Geometry check sheet. Reference: the model listing, model coordinates, mm. A direction names the side the tool comes from. Round coordinates to 2 decimals unless told otherwise and drop trailing zeros. Order: outer loops, then holes, each group sorted by start corner. A loop starts at its lowest first (then second) coordinate and runs counter-clockwise, first axis right, second up.
(1) Cross-section at A-A on z = 1.5. Enter the section's corners in (x, y), and give its area (3 significant figures).
(2) Cross-section at D-D on x = 0. Enter the section's corners in (y, z), and give its area (3 significant figures).
(3) Cross-section at C-C on z = -18.5. Enter the section's corners in (x, y), and give its area (3 significant figures).
(4) Gauge pin test, flat ends, axial feed: P1, Ø5, axis at x = 1, z = -5.5, coming from the -Y side; P2, Ø1.1, axis at x = -0.5, z = -30.5, coming from the -Y side; P3, Ø6.5, axis at x = 2, y = 3, coming from the -Z side; P4, Ø1, axis at x = 9.5, y = 4, coming from the +Z side. Record the tip position at first contact, or that the pin passes through.
(5) Thickness scan on L1, parallel to Y at x = 9.5, z = 1.5; L2, parallel to Z at x = -2.25, y = -10.5; L3, parallel to X at y = 0, z = 2. Record the ranges inside material, lowest first.
(6) Draft check along Y on faces 4 (the face through (0, -11.1, 2)), 5 (the face through (0, -7, 5)), 6 (the face through (-0.2, -11.6, -29.5)). Enter one of: pulls with the +Y half, pulls with the -Y half, needs draft (parallel to the pull), parting line crosses it, or undercut.
(7) Set-up check for faces 1 (the face through (-0.2, -11.1, -29.5)), 2 (the face through (-11.2, -1, 2)), 3 (the face through (-0.2, -12.1, -30.5)): record each of +Z, -Z, +X, -X, +Y, -Y from which the full face is reachable in a straight line by a thin tool's end or side.
(8) Cross-section at B-B on y = -1.5. Enter the section's corners in (x, z), and give its area (3 significant figures).
from build123d import *

# Parameters (mm, degrees)
F0_W       = 26.4
F0_H       = 16
F0_W_2     = 22.4
F0_H_2     = 12
F1_DEPTH   = 5
F3_DEPTH   = 32
F4_W       = 26.4
F4_H       = 2
F5_DEPTH   = 5.1
F6_W       = 26.4
F6_H       = 2
F7_DEPTH   = 2
F8_W       = 26.4
F8_H       = 2
F9_DEPTH   = 1
F11_DEPTH  = 26.401
F13_DEPTH  = 2
F14_DEPTH  = 26.4
F14_FACE_W = 22.4
F14_FACE_H = 6
F15_DEPTH  = 31.001
F16_DEPTH  = 25


with BuildPart() as f1:
    # F0 (on Top) → F1 (new body)
    with BuildSketch(Plane.XY):
        Rectangle(F0_W, F0_H)
        Rectangle(F0_W_2, F0_H_2, mode=Mode.SUBTRACT)
    extrude(amount=F1_DEPTH)

    # F2 (on face) → F3 (join)
    with BuildSketch(Plane(origin=(0, 0, 0), x_dir=(1, 0, 0), z_dir=(0, 0, -1))):
        Polygon((13.2, 8), (-13.2, 8), (-13.2, 6), (-11.2, 6), (11.2, 6), (13.2, 6), align=None)
    extrude(amount=F3_DEPTH)

    # F4 (on face) → F5 (join)
    with BuildSketch(Plane.XZ.offset(8)):
        with Locations((0, 4)):
            Rectangle(F4_W, F4_H)
        with Locations((0, -31)):
            Rectangle(F4_W, F4_H)
    extrude(amount=F5_DEPTH)

    # F6 (on face) → F7 (join)
    with BuildSketch(Plane(origin=(0, 0, 3), x_dir=(1, 0, 0), z_dir=(0, 0, -1))):
        with Locations((0, 12.1)):
            Rectangle(F6_W, F6_H)
    extrude(amount=F7_DEPTH)

    # F8 (on face) → F9 (join)
    with BuildSketch(Plane.XY.offset(-30)):
        with Locations((0, -12.1)):
            Rectangle(F8_W, F8_H)
    extrude(amount=F9_DEPTH)

    # F10 (on face) → F11 (cut, through all)
    with BuildSketch(Plane(origin=(-13.2, 0, 0), x_dir=(0, -1, 0), z_dir=(-1, 0, 0))):
        Polygon((11.1, -29), (12.1, -30), (12.1, -31), (6, -31), (6, -32), (13.1, -32), (13.1, -29), align=None)
    extrude(amount=-F11_DEPTH, mode=Mode.SUBTRACT)

    # F12 (on face) → F13 (join, through all)
    with BuildSketch(Plane(origin=(-13.2, 0, 0), x_dir=(0, -1, 0), z_dir=(-1, 0, 0))):
        Polygon((0, 0), (6, 0), (6, -7), (6, -31), (12.1, -31), (12.1, -30), (11.1, -29), (11.1, -30), (8, -30), (8, 3), (11.1, 3), (11.1, 1), (13.1, 1), (13.1, 5), (-8, 5), (-8, 0), align=None)
    extrude(amount=-F13_DEPTH)

    # F12 (on face) → F14 (join, through all)
    with BuildSketch(Plane(origin=(-13.2, 0, 0), x_dir=(0, -1, 0), z_dir=(-1, 0, 0))):
        Polygon((6, -7), (6, 0), (0, 0), align=None)
    extrude(amount=-F14_DEPTH)

    # F14_face (on face) → F15 (cut, through all)
    with BuildSketch(Plane(origin=(0, -3, 0), x_dir=(1, 0, 0), z_dir=(0, 0, 1))):
        Rectangle(F14_FACE_W, F14_FACE_H)
    extrude(amount=-F15_DEPTH, mode=Mode.SUBTRACT)

    # F4 (on face) → F16 (cut)
    with BuildSketch(Plane.XZ.offset(8)):
        with BuildLine():
            ThreePointArc((-10.2, -25.023081), (-9.448807, -27.008746), (-7.571423, -28))
            Line((-7.571423, -28), (7.2, -28))
            ThreePointArc((7.2, -28), (9.32132, -27.12132), (10.2, -25))
            Line((10.2, -25), (10.2, -17.8))
            ThreePointArc((10.2, -17.8), (0, -7.6), (-10.2, -17.8))
            Line((-10.2, -17.8), (-10.2, -25.023081))
        make_face()
    extrude(amount=-F16_DEPTH, mode=Mode.SUBTRACT)


solid = f1.part
Found:
1. outline: (-13.2, -13.1) - (13.2, -13.1) - (13.2, -11.1) - (-13.2, -11.1) - close; (-13.2, -8) - (13.2, -8) - (13.2, 8) - (-13.2, 8) - close; hole (-11.2, -6) - (11.2, -6) - (11.2, 6) - (-11.2, 6) - close
1. area: 206 mm2
2. outline: (-13.1, 1) - (-11.1, 1) - (-11.1, 3) - (-8, 3) - (-8, -7.6) - (-6, -7.6) - (-6, 5) - (-13.1, 5) - close; (-12.1, -31) - (-6, -31) - (-6, -28) - (-8, -28) - (-8, -30) - (-11.1, -30) - (-11.1, -29) - (-12.1, -30) - close; (6, 0) - (8, 0) - (8, 5) - (6, 5) - close
2. area: 60.0 mm2
3. outline: (-13.2, -8) - (-10.2, -8) - (-10.2, -6) - (-13.2, -6) - close; (10.2, -8) - (13.2, -8) - (13.2, -6) - (10.2, -6) - close
3. area: 12.0 mm2
4. P1: stops at y = -8
4. P2: stops at y = -12.1
4. P3: stops at z = 0
4. P4: passes through
5. L1: y = -13.1 to -11.1, -8 to -6, 6 to 8
5. L2: z = -31 to -30, 3 to 5
5. L3: x = -13.2 to -11.2, 11.2 to 13.2
6. face 4: undercut
6. face 5: needs draft
6. face 6: pulls with the -Y half
7. face 1: +X, -X
7. face 2: +Z, -Z
7. face 3: -Z, +X, -X, -Y
8. outline: (-13.2, -1.75) - (-11.2, -1.75) - (-11.2, 5) - (-13.2, 5) - close; (11.2, -1.75) - (13.2, -1.75) - (13.2, 5) - (11.2, 5) - close
8. area: 27.0 mm2
